Could you check a few things on this model? Use its own coordinates, in mm. A direction names the side the tool comes from. Give positions to 0.01 mm unless a question says otherwise; leave off trailing zeros. Loops run counter-clockwise (first coordinate to the right, second up) from the corner with the lowest first, then second, coordinate; pieces in that order, holes last.
1. For faces 1 (the cylindrical face through (63.89, 254.02, -1.69)), 2 (the flat face through (-1, 162, -15)), 3 (the flat face through (0, 100, 0)), 4 (the flat face through (36.5, 332, 0)), which set-ups out of +Z, -Z, +X, -X, +Y, -Y let a thin tool reach every point of the face, with its end or its side?
2. Imagine slicing it at A-A (x = 33). List the corners of the cut face in (y, z) for me, plus the area to 3 significant figures.
3. I need wall thicknesses on line 1 along Y through (x, z) = (-8.5, -6); line 2 along Z through (x, y) = (-37.25, 337.5); line 3 along Y through (x, z) = (45.5, -12.5). Which ranges of each line are inside material? Lowest first, please.
4. Imagine slicing it at C-C (y = 152). List the corners of the cut face in (x, z) for me, plus the area to 3 significant figures.
5. Imagine slicing it at D-D (y = 34.5). List the corners of the cut face in (x, z) for me, plus the area to 3 significant figures.
6. Imagine slicing it at B-B (y = 337.5). List the corners of the cut face in (x, z) for me, plus the area to 3 significant figures.
7. Thinking about a two-plate mould opening in Z: for faces 5 (the cylindrical face through (-10.74, 49.3, 2.38)), 6 (the flat face through (-9.3, 0, 6.2)), 7 (the cylindrical face through (64.094, 162.815, 12.719)), which applies, +Z half, -Z half, draft (parallel to the pull), parting line (faces both ways), or undercut?
8. For P1, Ø4, axis at x = -16.5, z = -12, coming from the -Y side; P2, Ø3, axis at y = 103.5, z = -9.5, coming from the +X side; P3, Ø3, axis at y = 229, z = 5, coming from the -X side; P4, Ø9, axis at y = 337.5, z = 0, coming from the +X side, each with a flat end and sliding along its axis, tell me the tip position at first contact or that it passes through.
```python
from build123d import *

# Parameters (mm, degrees)
SKETCH1_R               = 14
BOSS_EXTRUDE1_DEPTH     = 140
SKETCH2_W               = 133
SKETCH2_H               = 30
BOSS_EXTRUDE2_DEPTH     = 45
SKETCH3_R               = 13
BOSS_EXTRUDE3_DEPTH     = 140
FILLET1_R               = 8
BOSS_EXTRUDE4_START     = -10
SKETCH5_W               = 2.25
SKETCH5_H               = 23
BOSS_EXTRUDE4_DEPTH     = 35
CUT_EXTRUDE1_DEPTH      = 366.14928454
CUT_EXTRUDE1_DEPTH_BACK = 366.14928454
SKETCH6_R               = 5
BOSS_EXTRUDE5_START     = -140
BOSS_EXTRUDE5_DEPTH     = 2
CUT_EXTRUDE2_REACH      = 224.761
SKETCH9_R               = 1.5
SKETCH10_R              = 11
CUT_EXTRUDE3_DEPTH      = 100


with BuildPart() as part:
    # Sketch1 → Boss-Extrude1 (new body)
    with BuildSketch(Plane(origin=(0, 0, 0), x_dir=(1, 0, 0), z_dir=(0, 1, 0))):
        with Locations(Location((0, 0, 0), (0, 0, 270))):
            Circle(SKETCH1_R)
    extrude(amount=BOSS_EXTRUDE1_DEPTH)

    # Sketch2 → Boss-Extrude2 (add)
    with BuildSketch(Plane(origin=(0, 140, 0), x_dir=(1, 0, 0), z_dir=(0, 1, 0))):
        Rectangle(SKETCH2_W, SKETCH2_H)
    extrude(amount=BOSS_EXTRUDE2_DEPTH)

    # Sketch3 → Boss-Extrude3 (add)
    with BuildSketch(Plane(origin=(0, 185, 0), x_dir=(1, 0, 0), z_dir=(0, 1, 0))):
        with Locations(Location((-51, 0, 0), (0, 0, 270))):
            Circle(SKETCH3_R)
        with Locations(Location((51, 0, 0), (0, 0, 270))):
            Circle(SKETCH3_R)
    extrude(amount=BOSS_EXTRUDE3_DEPTH)

    # Fillet1
    fillet1_edges = [part.edges().sort_by_distance(p)[0] for p in [
        (-66.5, 162.5, 15),
        (66.5, 162.5, 15),
        (66.5, 162.5, -15),
        (-66.5, 162.5, -15),
    ]]
    fillet(fillet1_edges, radius=FILLET1_R)

    # Sketch5 → Boss-Extrude4 (add)
    with BuildSketch(Plane(origin=(0, 325, 0), x_dir=(1, 0, 0), z_dir=(0, 1, 0)).offset(BOSS_EXTRUDE4_START)):
        with Locations((-37.625, 0)):
            Rectangle(SKETCH5_W, SKETCH5_H)
        with Locations((37.625, 0)):
            Rectangle(SKETCH5_W, SKETCH5_H)
    extrude(amount=BOSS_EXTRUDE4_DEPTH)

    # Sketch6 → Cut-Extrude1 (cut, two sides: drawn at the far end of the back side and taken through both)
    with BuildSketch(Plane(origin=(-36.5, 0, 0), x_dir=(0, 0, -1), z_dir=(1, 0, 0)).offset(-CUT_EXTRUDE1_DEPTH_BACK)):
        with Locations((0, 337.5)):
            Circle(SKETCH6_R)
    extrude(amount=CUT_EXTRUDE1_DEPTH + CUT_EXTRUDE1_DEPTH_BACK, mode=Mode.SUBTRACT)

    # Sketch8 → Boss-Extrude5 (add)
    with BuildSketch(Plane(origin=(0, 350, 0), x_dir=(1, 0, 0), z_dir=(0, 1, 0)).offset(BOSS_EXTRUDE5_START)):
        Polygon((17.5, 16), (-17.5, 16), (-49.5, 16), (-49.5, 12), (-17.5, 12), (-17.5, -12), (-49.5, -12), (-49.5, -16), (-17.5, -16), (17.5, -16), (49.5, -16), (49.5, -12), (17.5, -12), (17.5, 12), (49.5, 12), (49.5, 16), align=None)
    extrude(amount=BOSS_EXTRUDE5_DEPTH)

    # Sketch9 → Cut-Extrude2 (cut, up to next)
    with BuildSketch(Plane(origin=(0, 212, 0), x_dir=(1, 0, 0), z_dir=(0, 1, 0)), mode=Mode.PRIVATE) as cut_extrude2_sk1:
        with Locations(Location((0, 0, 0), (0, 0, 270))):
            Circle(SKETCH9_R)
    cut_extrude2_tool1 = extrude(cut_extrude2_sk1.sketch, amount=-CUT_EXTRUDE2_REACH, mode=Mode.PRIVATE) & part.part
    add(cut_extrude2_tool1.solids().sort_by_distance((0, 212, 0))[0], mode=Mode.SUBTRACT)

    # Sketch10 → Cut-Extrude3 (cut)
    with BuildSketch(Plane.XZ):
        with Locations(Location((0, 0, 0), (0, 0, 270))):
            Circle(SKETCH10_R)
    extrude(amount=-CUT_EXTRUDE3_DEPTH, mode=Mode.SUBTRACT)


solid = part.part
```
Derived:
1. face 1: none
1. face 2: -Z, +X, -X, -Y
1. face 3: -Y
1. face 4: +Z, -Z, +Y
2. outline: (140, -15) - (185, -15) - (185, 15) - (140, 15) - close; (210, -16) - (212, -16) - (212, -12) - (210, -12) - close; (210, 12) - (212, 12) - (212, 16) - (210, 16) - close
2. area: 1,370 mm2
3. line 1: y = 100 to 185, 210 to 212
3. line 2: z = -11.5 to -5, 5 to 11.5
3. line 3: y = 140 to 185, 210 to 212
4. outline: (-66.5, -7) arc R8 ccw to (-58.5, -15) - (58.5, -15) arc R8 ccw to (66.5, -7) - (66.5, 7) arc R8 ccw to (58.5, 15) - (-58.5, 15) arc R8 ccw to (-66.5, 7) - close
4. area: 3,940 mm2
5. outline: circle Ø28 at (0, 0); hole circle Ø22 at (0, 0)
5. area: 236 mm2
6. outline: (-38.75, -11.5) - (-36.5, -11.5) - (-36.5, -5) - (-38.75, -5) - close; (-38.75, 5) - (-36.5, 5) - (-36.5, 11.5) - (-38.75, 11.5) - close; (36.5, -11.5) - (38.75, -11.5) - (38.75, -5) - (36.5, -5) - close; (36.5, 5) - (38.75, 5) - (38.75, 11.5) - (36.5, 11.5) - close
6. area: 58.5 mm2
7. face 5: undercut
7. face 6: draft
7. face 7: +Z half
8. P1: stops at y = 140
8. P2: stops at x = 11.49
8. P3: stops at x = -63.52
8. P4: passes through
